The listing builds one solid part. Answer for the finished solid, in the listing's coordinates (mm). Round coordinates to 2 decimals unless told otherwise and drop trailing zeros. Write each loop counter-clockwise with the first axis right and the second up, starting at its lowest first coordinate (ties: lowest second). Pieces come first, ordered by that corner, then holes. Notation, with made-up numbers: M 87,76 L 123,76 A6 cw 123,85 Z; hole C 20,-31.5 d1. An arc over 180 degrees is marked long. One line per item, written item: value. Start each with the question number.
(1) Consider probe 1 along Y at (x, z) = (5.5, -42.5); probe 2 along Z at (x, y) = (0.75, -3); probe 3 along Z at (x, y) = (1.5, -22). Determine where each line is inside the solid, lowest interval first.
(2) For a pull along Z with two mould halves and no side action, classify faces 1 (the cylindrical face through (3.22, -41.88, -15.86)), 2 (the flat face through (6.35, -16, 16)), 3 (the flat face through (3, -3, 78.435)), 4 (the cylindrical face through (3.131, -47.267, 34.266)) as released by +Z, released by -Z, zero draft, split by the parting line, or undercut.
(3) Section C-C (y = -38) is taken. Determine the outline of the cut face in (x, z).
(4) Given P1, Ø5, axis at y = -23.13, z = 72.08, coming from the -X side; P2, Ø2.5, axis at y = -48.53, z = -42.22, coming from the +X side, each flat-ended and moving along its own axis, determine where each tip first touches the part or whether it passes through.
(5) Section B-B (x = 3) is taken. State how many separate pieces and enclosed holes the cut face has, plus the area to 3 significant figures.
(6) Section A-A (z = -7.5) is taken. Determine the outline of the cut face in (x, y), plus the area to 3 significant figures.
Autodesk Inventor part; units mm, degrees
ref_plane "YZ Plane" through (0, 0, 0) normal (1, 0, 0) x (0, 1, 0)
ref_plane "XZ Plane" through (0, 0, 0) normal (0, 1, 0) x (-1, 0, 0)
ref_plane "XY Plane" through (0, 0, 0) normal (0, 0, 1) x (1, 0, 0)
sketch "Sketch1" plane through (0, 0, 0) normal (1, 0, 0) x (0, 1, 0)
  line L0 (46.7204, 78.4349) -> (-54.8796, 78.4349)
  line L1 (-54.8796, 78.4349) -> (-54.8796, -48.5651)
  line L2 (-54.8796, -48.5651) -> (46.7204, -48.5651)
  line L3 (46.7204, -48.5651) -> (46.7204, 78.4349)
  point P0 (0, 0)
  dimension "d0" = 127
  dimension "d1" = 101.6
extrude "Extrusion1" add sketch "Sketch1" along normal blind 6.35
sketch "Sketch2" plane through (6.35, 0, 0) normal (1, 0, 0) x (0, 0, -1)
  line L0 (48.5651, 46.7204) -> (-78.4349, 46.7204)
  line L1 (-78.4349, 46.7204) -> (-78.4349, -54.8796)
  line L2 (-78.4349, -54.8796) -> (48.5651, -54.8796)
  line L3 (48.5651, -54.8796) -> (48.5651, 46.7204)
  point P0 (0, 0)
  point P1 (-72.0849, 40.3704)
  point P2 (42.2151, 40.3704)
  point P3 (42.2151, -48.5296)
  point P4 (-72.0849, -48.5296)
  dimension "d4" = 0
  dimension "d5" = 0
  dimension "d6" = 0
  dimension "d7" = 0
  dimension "d8" = 6.35
  dimension "d9" = 6.35
  dimension "d10" = 6.35
  dimension "d11" = 6.35
hole "Hole1" at (6.35, 40.3704, 72.0849) at (6.35, 40.3704, -42.2151) at (6.35, -48.5296, -42.2151) at (6.35, -48.5296, 72.0849) direction (-1, 0, 0) diameter 4.318 end through all
sketch "Sketch3" plane through (6.35, 0, 0) normal (1, 0, 0) x (0, 0, -1)
  circle A0 centre (-46.6849, -23.1296) radius 9.652
  line L0 (-78.4349, -54.8796) -> (48.5651, -54.8796)
  line L1 (-78.4349, 46.7204) -> (-78.4349, -54.8796)
  point P0 (0, 0)
  dimension "d19" = 19.304
  dimension "d20" = 31.75
  dimension "d21" = 31.75
extrude "Extrusion2" cut sketch "Sketch3" against normal blind 61.9125
sketch "Sketch4" plane through (6.35, 0, 0) normal (1, 0, 0) x (0, 0, -1)
  circle A0 centre (-46.6849, -23.1296) radius 9.652
  circle A1 centre (-46.6849, -23.1296) radius 9.652
  circle A2 centre (-46.6849, -23.1296) radius 25.4
  line L0 (-46.6849, -23.1296) -> (-105.0514, -23.1296)
  line L1 (-46.6849, -23.1296) -> (-64.9089, 8.4353)
  line L2 (-46.6849, -23.1296) -> (-26.8908, 11.1548)
  line L3 (-46.6849, -23.1296) -> (1.7612, -23.1296)
  line L4 (-46.6849, -23.1296) -> (-29.0867, -53.6105)
  line L5 (-46.6849, -23.1296) -> (-67.8043, -59.7094)
  point P0 (0, 0)
  point P1 (-72.0849, -23.1296)
  point P2 (-21.2849, -23.1296)
  point P3 (-59.3849, -1.1326)
  point P4 (-33.9849, -1.1326)
  point P5 (-33.9849, -45.1267)
  point P6 (-59.3849, -45.1267)
  dimension "d24" = 50.8
  dimension "d25" = 60
  dimension "d26" = 60
  dimension "d27" = 60
  dimension "d28" = 60
hole "Hole2" at (6.35, -23.1296, 72.0849) at (6.35, -23.1296, 21.2849) at (6.35, -1.1326, 59.3849) at (6.35, -1.1326, 33.9849) at (6.35, -45.1267, 33.9849) at (6.35, -45.1267, 59.3849) direction (-1, 0, 0) diameter 4.318 end through all
sketch "Sketch5" plane through (6.35, 0, 0) normal (1, 0, 0) x (0, 0, -1)
  circle A0 centre (-14.6316, -0.2696) radius 11.1125
  circle A1 centre (-46.6849, -23.1296) radius 9.652
  circle A2 centre (-46.6849, -23.1296) radius 39.37
  point P0 (0, 0)
  dimension "d37" = 78.74
  dimension "d36" = 22.225
  dimension "d44" = 22.86
extrude "Extrusion3" cut sketch "Sketch5" against normal blind 66.675 contours A0 A2 | A2 A0 picked at (-11.8926, 2.0476) picked at (-17.7425, -2.4882)
sketch "Sketch6" plane through (6.35, 0, 0) normal (1, 0, 0) x (0, 0, -1)
  circle A0 centre (-14.6316, -0.2696) radius 11.1125
  circle A1 centre (-14.6316, -0.2696) radius 40.64
  circle A2 centre (10.7367, -32.0196) radius 11.1125
  line L0 (48.5651, 46.7204) -> (-78.4349, 46.7204)
  point P0 (0, 0)
  dimension "d43" = 81.28
  dimension "d40" = 22.225
  dimension "d76" = 78.74
extrude "Extrusion4" cut sketch "Sketch6" against normal blind 39.6875 contours A2 A1 | A1 A2 picked at (8.3538, -29.0373) picked at (12.8293, -34.938)
properties part number "InsideMotorPlate" material "Aluminum 6061"
Recorded:
1. probe 1: y = -54.88 to -50.67, -46.39 to 38.23, 42.51 to 46.72
1. probe 2: z = -48.57 to 3.86, 25.4 to 32.9, 35.07 to 58.3, 60.47 to 78.43
1. probe 3: z = -48.57 to -15.54, -5.93 to 19.44, 23.12 to 37.1, 56.27 to 70.24, 73.92 to 78.43
2. face 1: undercut
2. face 2: zero draft
2. face 3: released by +Z
2. face 4: undercut
3. outline: M 0,-48.57 L 6.35,-48.57 L 6.35,-20.1 L 0,-20.1 Z; M 0,-1.37 L 6.35,-1.37 L 6.35,78.43 L 0,78.43 Z
4. P1: stops at x = 0
4. P2: passes through
5. separate pieces: 1
5. enclosed holes: 13
5. area: 11,700 mm2
6. outline: M 0,-54.88 L 6.35,-54.88 L 6.35,-42.65 L 0,-42.65 Z; M 0,-21.39 L 6.35,-21.39 L 6.35,46.72 L 0,46.72 Z
6. area: 510 mm2
